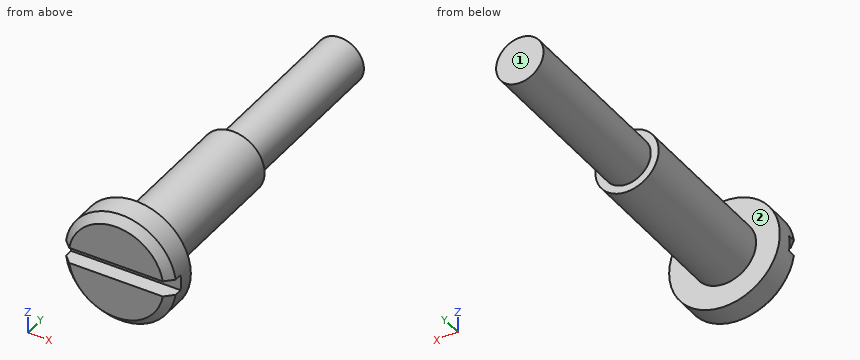
```python
from build123d import *

# Parameters (mm, degrees)
F0_R          = 3
F1_DEPTH      = 22
F1_DEPTH_BACK = 24
F0_R_2        = 4
F2_DEPTH      = 24
F3_START      = 20
F0_R_3        = 7
F3_DEPTH      = 4
F5_START      = 22
F4_W          = 30
F4_H          = 2
F5_DEPTH      = 3
F6_SIZE       = 1


with BuildPart() as f1:
    # F0 (on Front) → F1 (new body, two sides)
    with BuildSketch(Plane.XZ) as f1_sk:
        Circle(F0_R)
    extrude(amount=-F1_DEPTH)
    extrude(f1_sk.sketch, amount=F1_DEPTH_BACK)

    # F0 (on Front) → F2 (join)
    with BuildSketch(Plane.XZ):
        Circle(F0_R_2)
        Circle(F0_R, mode=Mode.SUBTRACT)
    extrude(amount=F2_DEPTH)

    # F0 (on Front) → F3 (join)
    with BuildSketch(Plane.XZ.offset(F3_START)):
        Circle(F0_R_3)
        Circle(F0_R_2, mode=Mode.SUBTRACT)
    extrude(amount=F3_DEPTH)

    # F4 (on Front) → F5 (cut)
    with BuildSketch(Plane.XZ.offset(F5_START)):
        Rectangle(F4_W, F4_H)
    extrude(amount=F5_DEPTH, mode=Mode.SUBTRACT)

    # F6
    f6_edges = [f1.edges().sort_by_distance(p)[0] for p in [
        (0, -24, 7),
        (0, -24, -7),
    ]]
    chamfer(f6_edges, length=F6_SIZE)


solid = f1.part
```
Here's how the part is built. I have some questions about the finished solid (model axes, mm). Face numbers are marked on the shaded views. A direction names the side the tool comes from. Give positions to 0.01 mm unless a question says otherwise; leave off trailing zeros. Order: outer loops, then holes, each group sorted by start corner. A loop starts at its lowest first (then second) coordinate and runs counter-clockwise, first axis right, second up. Notation, with made-up numbers: M -22.5,44.25 L 33.5,44.25 A14 ccw 33.5,61.25 Z; hole C -4,81.5 d4. An arc over 180 degrees is marked long. Use a Markdown table: item, result. Add a question column.
1. On a 3-axis mill with a long thin cutter (end or side, diameter ignored), from which of +Z, -Z, +X, -X, +Y, -Y can I reach the whole of each face in a straight line? I mean the marked faces 1 and 2. Say none if no direction works.
2. Suppose I cut it at B-B (z = 0). List the corners of the cut face in (x, y) for me.
3. Suppose I cut it at C-C (y = 4.5). List the corners of the cut face in (x, z) for me, and give its area (3 significant figures).
4. Suppose I cut it at A-A (x = 0). List the corners of the cut face in (y, z) for me.
5. I need wall thicknesses on probe 1 along Y at (x, z) = (1.75, 4); probe 2 along Y at (x, z) = (-1.5, 3); probe 3 along Z at (x, y) = (2.5, 19.5). Which ranges of each line are inside material? Lowest first, please. Write a range as from..to.
6. For pin 1 Ø0.6 at (x, y) = (0, -23.5) entering from -Z; pin 2 Ø0.6 at (x, z) = (0.5, 0.5) entering from -Y; pin 3 Ø2 at (x, y) = (5.5, -18.5) entering from -Z; pin 4 Ø4 at (x, y) = (3.5, 15) entering from +Z, each with a flat end and sliding along its axis, tell me the tip position at first contact or that it passes through.
Results list:
| question | item | result |
|---|---|---|
| 1 | face 1 | +Z, -Z, +X, -X, +Y |
| 1 | face 2 | +Y |
| 2 | outline | M -7,-22 L 7,-22 L 7,-20 L 4,-20 L 4,0 L 3,0 L 3,22 L -3,22 L -3,0 L -4,0 L -4,-20 L -7,-20 Z |
| 3 | outline | C 0,0 d6 |
| 3 | area | 28.3 mm² |
| 4 | outline | M -24,-6 L -23,-7 L -20,-7 L -20,-4 L 0,-4 L 0,-3 L 22,-3 L 22,3 L 0,3 L 0,4 L -20,4 L -20,7 L -23,7 L -24,6 L -24,1 L -22,1 L -22,-1 L -24,-1 Z |
| 5 | probe 1 | y = -24..-20 |
| 5 | probe 2 | y = -24..0 |
| 5 | probe 3 | z = -1.66..1.66 |
| 6 | pin 1 | stops at z = -6.8 |
| 6 | pin 2 | stops at y = -22 |
| 6 | pin 3 | passes through |
| 6 | pin 4 | stops at z = 2.6 |
